Can you work these out from the drawing? Everything is in mm from the part's minimum corner. A direction names the side the tool comes from. Round coordinates to 2 decimals unless told otherwise and drop trailing zeros. Order: outer loops, then holes, each group sorted by start corner. A loop starts at its lowest first (then second) coordinate and runs counter-clockwise, first axis right, second up. Notation, with made-up numbers: (-4, 87.25) -> (20, 87.25) arc R21 cw to (20, 113.25) -> close; hole circle Ø3 at (58.5, -18.5). An arc over 180 degrees is marked (long way). One line per item, written item: value.
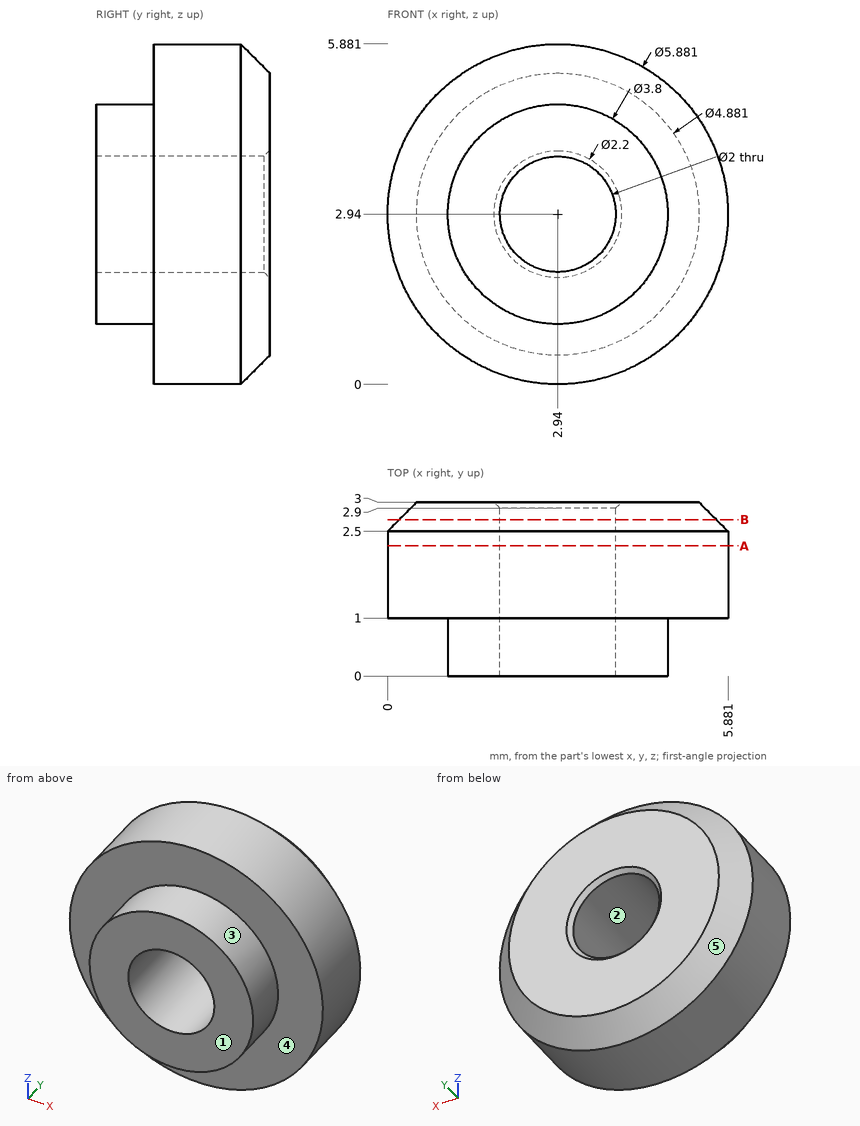
Q1. On a 3-axis mill with a long thin cutter (end or side, diameter ignored), from which of +Z, -Z, +X, -X, +Y, -Y can I reach the whole of each face in a straight line? I mean the marked faces 4 and 5. Say none if no direction works.
Answers below:
face 4: -Y
face 5: +Y
Q2. Will these pins go through, and if not, where does the flat tip stop? pin 1 Ø1.2 at (x, z) = (2.94, 2.94) entering from +Y; pin 2 Ø3 at (x, z) = (2.5, 3.5) entering from -Y.
Answers below:
pin 1: through
pin 2: y = 0
Q3. Please list where these lines run through material, in increasing order: line 1 along X through (y, z) = (0.45, 2.9); line 2 along Y through (x, z) = (2.55, 0.6); line 3 along Z through (x, y) = (3, 1.45).
Answers below:
line 1: 1.04 to 1.94, 3.94 to 4.84
line 2: 1 to 3
line 3: 0 to 1.94, 3.94 to 5.88
Q4. We'd pull the mould along Z, two halves only. Please class the marked faces 1, 2 and 3: released by +Z, released by -Z, zero draft, split by the parting line, or undercut.
Answers below:
face 1: zero draft
face 2: undercut
face 3: split by the parting line
Q5. I want a section at B-B on y = 2.7. List the corners of the cut face in (x, z) for me.
Answers below:
outline: circle Ø5.48 at (2.94, 2.94); hole circle Ø2 at (2.94, 2.94)
Q6. I want a section at A-A on y = 2.25. List the corners of the cut face in (x, z) for me, plus the area to 3 significant figures.
Answers below:
outline: circle Ø5.88 at (2.94, 2.94); hole circle Ø2 at (2.94, 2.94)
area: 24.0 mm^2
